```python
from build123d import *

# Parameters (mm, degrees)
SKETCH1_R                 = 20
BOSS_EXTRUDE1_DEPTH       = 2
SKETCH4_R                 = 20.15
BOSS_EXTRUDE3_DEPTH       = 33
SKETCH5_R                 = 10
BOSS_EXTRUDE4_DEPTH       = 5
BOSS_EXTRUDE5_DEPTH       = 13
FILLET2_R                 = 0.5
FILLET3_R                 = 1.5
M3X0_5_TAPPED_HOLE1_D     = 2.5
M3X0_5_TAPPED_HOLE1_DEPTH = 5.5
M3X0_5_TAPPED_HOLE1_TIP   = 0.751075774


with BuildPart() as part:
    # Sketch1 → Boss-Extrude1 (new body)
    with BuildSketch(Plane(origin=(0, 0, 0), x_dir=(1, 0, 0), z_dir=(0, 1, 0))):
        with Locations(Location((0, 0, 0), (0, 0, 270))):
            Circle(SKETCH1_R)
    extrude(amount=-BOSS_EXTRUDE1_DEPTH)

    # Sketch4 → Boss-Extrude3 (add)
    with BuildSketch(Plane.XZ.offset(2)):
        with Locations(Location((0, 0, 0), (0, 0, 270))):
            Circle(SKETCH4_R)
    extrude(amount=BOSS_EXTRUDE3_DEPTH)

    # Sketch5 → Boss-Extrude4 (add)
    with BuildSketch(Plane(origin=(0, 0, 0), x_dir=(1, 0, 0), z_dir=(0, 1, 0))):
        with Locations(Location((0, 0, 0), (0, 0, 270))):
            Circle(SKETCH5_R)
    extrude(amount=BOSS_EXTRUDE4_DEPTH)

    # Sketch7 → Boss-Extrude5 (add)
    with BuildSketch(Plane(origin=(0, 5, 0), x_dir=(1, 0, 0), z_dir=(0, 1, 0))):
        with BuildLine():
            Line((-1.658312395, -2.5), (1.658312395, -2.5))
            ThreePointArc((1.658312395, -2.5), (0, 3), (-1.658312395, -2.5))
        make_face()
    extrude(amount=BOSS_EXTRUDE5_DEPTH)

    # Fillet2
    # the kernel refuses this fillet: 0.5 mm, written as the material it takes off along each edge
    with BuildSketch(Plane(origin=(0, 5, 0), x_dir=(0, 0, 1), z_dir=(-1, 0, 0))) as fillet2_piece_1:
        with BuildLine():
            CenterArc((10 - FILLET2_R, -FILLET2_R), FILLET2_R, 0, 90)
            Line((10 - FILLET2_R, 0), (10 - FILLET2_R, FILLET2_R * 0.02))
            Line((10 - FILLET2_R, FILLET2_R * 0.02), (10 + FILLET2_R * 0.02, FILLET2_R * 0.02))
            Line((10 + FILLET2_R * 0.02, FILLET2_R * 0.02), (10 + FILLET2_R * 0.02, -FILLET2_R))
            Line((10 + FILLET2_R * 0.02, -FILLET2_R), (10, -FILLET2_R))
        make_face()
    revolve(axis=Axis((0, 5, 0), (0, 1, 0)), mode=Mode.SUBTRACT)
    with BuildSketch(Plane(origin=(0, 0, 0), x_dir=(0, 0, 1), z_dir=(-1, 0, 0))) as fillet2_piece_2:
        with BuildLine():
            CenterArc((20 - FILLET2_R, -FILLET2_R), FILLET2_R, 0, 90)
            Line((20 - FILLET2_R, 0), (20 - FILLET2_R, FILLET2_R * 0.02))
            Line((20 - FILLET2_R, FILLET2_R * 0.02), (20 + FILLET2_R * 0.02, FILLET2_R * 0.02))
            Line((20 + FILLET2_R * 0.02, FILLET2_R * 0.02), (20 + FILLET2_R * 0.02, -FILLET2_R))
            Line((20 + FILLET2_R * 0.02, -FILLET2_R), (20, -FILLET2_R))
        make_face()
    revolve(axis=Axis((0, 0, 0), (0, 1, 0)), mode=Mode.SUBTRACT)
    with BuildSketch(Plane(origin=(0, -2, 0), x_dir=(0, 0, -1), z_dir=(-1, 0, 0))) as fillet2_piece_3:
        with BuildLine():
            CenterArc((19.65, 0.357071421), FILLET2_R, 314.427004001, 45.572995999)
            Line((20, 0), (20.007, -0.007141428))
            ThreePointArc((20.007, -0.007141428), (20.075, -0.01), (20.15, -0.01))
            Line((20.15, -0.01), (20.16, 0))
            Line((20.16, 0), (20.16, 0.357071421))
            Line((20.16, 0.357071421), (20.15, 0.357071421))
        make_face()
    revolve(axis=Axis((0, -2, 0), (0, -1, 0)), mode=Mode.SUBTRACT)

    # Fillet3
    fillet3_edges = [part.edges().sort_by_distance(p)[0] for p in [
        (0, -35, 20.15),
    ]]
    fillet(fillet3_edges, radius=FILLET3_R)

    # M3x0.5 Tapped Hole1
    with Locations(Plane(origin=(0, 0, 0), x_dir=(1, 0, 0), z_dir=(0, 1, 0))):
        with Locations((0, 15), (12.990381057, -7.5), (-12.990381057, -7.5)):
            Hole(M3X0_5_TAPPED_HOLE1_D / 2, depth=M3X0_5_TAPPED_HOLE1_DEPTH)
            with Locations((0, 0, -(M3X0_5_TAPPED_HOLE1_DEPTH + M3X0_5_TAPPED_HOLE1_TIP / 2))):  # 118° drill point
                Cone(0, M3X0_5_TAPPED_HOLE1_D / 2, M3X0_5_TAPPED_HOLE1_TIP, mode=Mode.SUBTRACT)


solid = part.part
```
Here's how the part is built. I have some questions about the finished solid (model axes, mm). A direction names the side the tool comes from. Coordinates: 2 decimals unless noted, no trailing zeros. Order: outer loops, then holes, each group sorted by start corner. A loop starts at its lowest first (then second) coordinate and runs counter-clockwise, first axis right, second up.
1) Will these pins go through, and if not, where does the flat tip stop? pin 1 (6 mm diameter, centred on x = 5, y = -7, fed in from +Z); pin 2 (12 mm diameter, centred on y = -7, z = -11, fed in from +X); pin 3 (11.5 mm diameter, centred on x = 5.5, z = -2, fed in from +Y); pin 4 (4 mm diameter, centred on x = 12.99, z = 7.5, fed in from +Y).
2) We'd pull the mould along Z, two halves only. Please class faces 3 (the face through (-0.05, -6.12, -14.79)), 4 (the face through (0, 11, 2.5)), 5 (the face through (5, 0, -9)): +Z half, -Z half, draft (parallel to the pull), parting line (faces both ways), or undercut.
3) I need wall thicknesses on line 1 (X direction, y = -1, z = 7) (3 decimals); line 2 (Y direction, x = -9.5, z = -8); line 3 (X direction, y = -3, z = 7). Which ranges of each line are inside material? Lowest first, please.
4) Imagine slicing it at A-A on z = 0. List the corners of the cut face in (x, y) for me, and give its area (3 significant figures).
5) Which directions (+Z, -Z, +X, -X, +Y, -Y) give clear straight access to the entire face, cutting with the end or side of a thin tool? Please do faces 1 (the face through (0, -35, 0)), 2 (the face through (0, 11, -3)).
6) Imagine slicing it at C-C on y = 13.5. List the corners of the cut face in (x, z) for me, and give its area (3 significant figures).
7) Imagine slicing it at B-B on y = -21. List the corners of the cut face in (x, z) for me, and give its area (3 significant figures).
Response values:
1. pin 1: stops at z = 20.05
1. pin 2: stops at x = 19.52
1. pin 3: stops at y = 18
1. pin 4: stops at y = 0
2. face 3: undercut
2. face 4: +Z half
2. face 5: draft
3. line 1: x = -18.735 to -14.136, -11.845 to 11.845, 14.136 to 18.735
3. line 2: y = -35 to 0
3. line 3: x = -18.9 to -14.14, -11.84 to 11.84, 14.14 to 18.9
4. outline: (-20.15, -33.5) arc R1.5 ccw to (-18.65, -35) - (18.65, -35) arc R1.5 ccw to (20.15, -33.5) - (20.15, -2.36) arc R0.5 ccw to (20, -2) - (20, -0.5) arc R0.5 ccw to (19.5, 0) - (10, 0) - (10, 4.5) arc R0.5 ccw to (9.5, 5) - (3, 5) - (3, 18) - (-3, 18) - (-3, 5) - (-9.5, 5) arc R0.5 ccw to (-10, 4.5) - (-10, 0) - (-19.5, 0) arc R0.5 ccw to (-20, -0.5) - (-20, -2) arc R0.5 ccw to (-20.15, -2.36) - close
4. area: 1,590 mm2
5. face 1: +Z, -Z, +X, -X, -Y
5. face 2: +Y
6. outline: (-1.66, 2.5) arc R3 ccw (long way) to (1.66, 2.5) - close
6. area: 27.1 mm2
7. outline: circle Ø40.3 at (0, 0)
7. area: 1,280 mm2
